Work out the finished part from the listing and answer in its coordinate system (mm). Coordinates: 2 decimals unless noted, no trailing zeros. Write each loop counter-clockwise with the first axis right and the second up, starting at its lowest first coordinate (ties: lowest second). Pieces come first, ordered by that corner, then holes. Notation, with made-up numbers: (1, 22.5) - (25, 22.5) arc R22 ccw to (25, 59.5) - close; hole circle Ø7 at (17, -40). An arc over 180 degrees is marked (long way). Use one line per item in the form item = value. Start each with the question number.
Item 1: A cutting plane is placed at B-B (y = 0). Write down the section's boundary in (x, z), then the cut area to 3 significant figures.
Item 2: A cutting plane is placed at C-C (z = 229). Write down the section's boundary in (x, y).
Item 3: Determine the mould class of faces 1 (the cylindrical face through (-1.08, -4.88, 197.2)), 2 (the cylindrical face through (-0.867, -3.905, 197.2)) for opening direction X: released by +X, released by -X, zero draft, split by the parting line, or undercut.
Item 4: Consider probe 1 along Y at (x, z) = (0, 168.5); probe 2 along Y at (x, z) = (0.75, 210); probe 3 along X at (y, z) = (-1, 253). Determine where each line is inside the solid, lowest interval first.
Item 5: A cutting plane is placed at A-A (x = 0). Write down the section's boundary in (y, z), then the cut area to 3 significant figures.
Item 6: Given pin 1 (1.8 mm diameter, centred on x = 0, z = 355, fed in from +Y); pin 2 (5 mm diameter, centred on x = 0, y = 0, fed in from +Z), each flat-ended and moving along its own axis, determine where each tip first touches the part or whether it passes through.
from build123d import *

# Parameters (mm, degrees)
SKETCH_1_R          = 5
SKETCH_1_R_2        = 4
EXTRUDE_1_DEPTH     = 400
SKETCH_2_R          = 1.5
CUT_EXTRUDE_1_DEPTH = 401.062495118
SKETCH_3_R          = 1.5
CUT_EXTRUDE_2_DEPTH = 401.06249522


with BuildPart() as part:
    # 草图1 → 凸台-拉伸1 (new body)
    with BuildSketch(Plane.XY):
        Circle(SKETCH_1_R)
        Circle(SKETCH_1_R_2, mode=Mode.SUBTRACT)
    extrude(amount=EXTRUDE_1_DEPTH)

    # 草图2 → 切除-拉伸1 (cut, through all)
    with BuildSketch(Plane(origin=(0, 0, 0), x_dir=(1, 0, 0), z_dir=(0, 1, 0))):
        with Locations(Location((0, -31.334408431, 0), (0, 0, 270))):
            Circle(SKETCH_2_R)
    extrude(amount=-CUT_EXTRUDE_1_DEPTH, mode=Mode.SUBTRACT)

    # 草图3 → 切除-拉伸2 (cut, through all)
    with BuildSketch(Plane(origin=(0, 0, 0), x_dir=(1, 0, 0), z_dir=(0, 1, 0))):
        with Locations(Location((0, -355, 0), (0, 0, 90))):
            Circle(SKETCH_3_R)
    extrude(amount=CUT_EXTRUDE_2_DEPTH, mode=Mode.SUBTRACT)


solid = part.part
Answer:
q1.outline = (-5, 0) - (-4, 0) - (-4, 400) - (-5, 400) - close; (4, 0) - (5, 0) - (5, 400) - (4, 400) - close
q1.area = 800 mm²
q2.outline = circle Ø10 at (0, 0); hole circle Ø8 at (0, 0)
q3.face_1 = split by the parting line
q3.face_2 = undercut
q4.probe_1 = -5 to -4, 4 to 5
q4.probe_2 = -4.94 to -3.93, 3.93 to 4.94
q4.probe_3 = -4.9 to -3.87, 3.87 to 4.9
q5.outline = (-5, 0) - (-4, 0) - (-4, 29.83) - (-5, 29.83) - close; (-5, 32.83) - (-4, 32.83) - (-4, 400) - (-5, 400) - close; (4, 0) - (5, 0) - (5, 353.5) - (4, 353.5) - close; (4, 356.5) - (5, 356.5) - (5, 400) - (4, 400) - close
q5.area = 794 mm²
q6.pin_1 = -3.9
q6.pin_2 = through
